Answer from the drawing. Dimensions are ordinates in mm from the lowest x, y and z of the part. A direction names the side the tool comes from. Coordinates: 2 decimals unless noted, no trailing zeros. Loops run counter-clockwise (first coordinate to the right, second up) from the corner with the lowest first, then second, coordinate; pieces in that order, holes last. Notation, with made-up numbers: M 32,44 L 66,44 A16 cw 66,48 Z; hole C 3.25,23.25 d11. An arc over 180 degrees is marked long. Put each result on its own line as item: value.
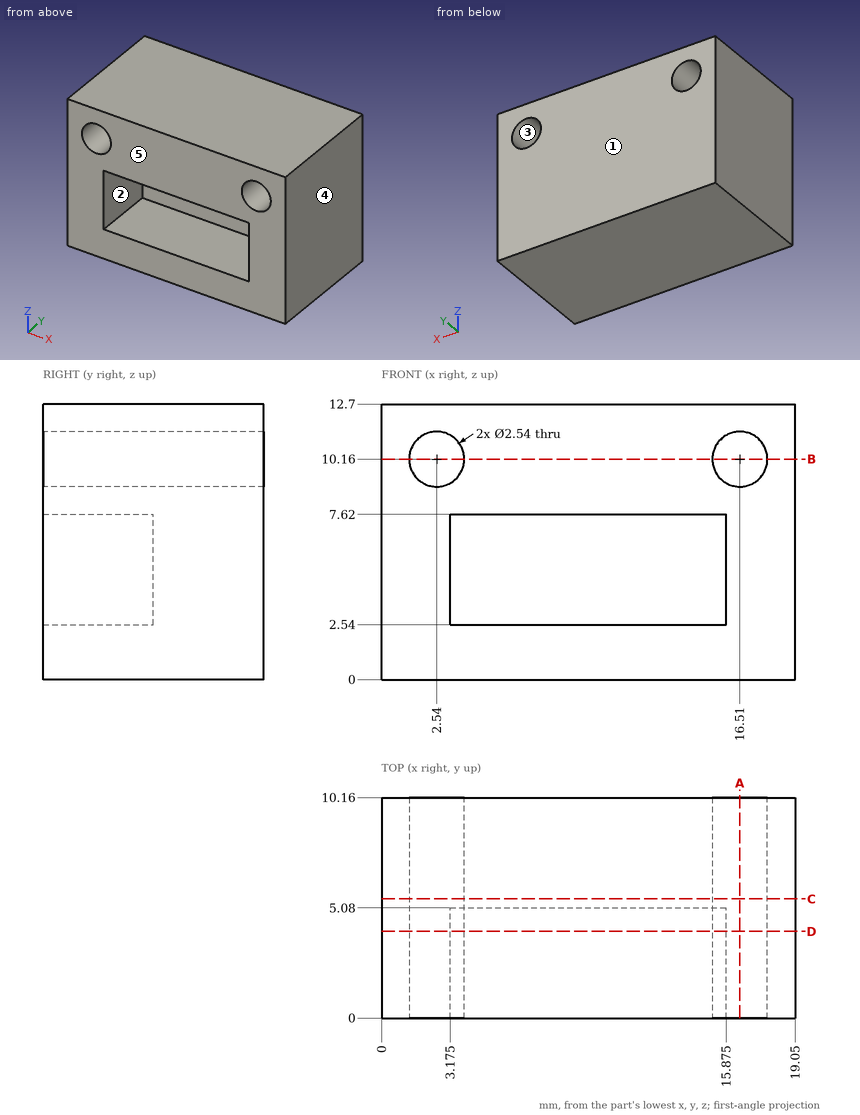
1) Which of the six approach directions +Z, -Z, +X, -X, +Y, -Y give full straight-line access (tool end or side, diameter ignored) to the marked faces 1 and 2?
Answer list:
face 1: +Z, -Z, +X, -X, +Y
face 2: -Y
2) Given pin 1 Ø1.5 at (x, z) = (9, 6) entering from -Y, flat-ended and moving along its own axis, determine where the tip first touches the part or whether it passes through.
Answer list:
pin 1: stops at y = 5.08
3) Find section B-B, the plane z = 10.16. Write down the section's boundary in (x, y), plus the area to 3 significant figures.
Answer list:
outline: M 0,0 L 1.27,0 L 1.27,10.16 L 0,10.16 Z; M 3.81,0 L 15.24,0 L 15.24,10.16 L 3.81,10.16 Z; M 17.78,0 L 19.05,0 L 19.05,10.16 L 17.78,10.16 Z
area: 142 mm^2
4) Find section A-A, the plane x = 16.51. Write down the section's boundary in (y, z), plus the area to 3 significant figures.
Answer list:
outline: M 0,0 L 10.16,0 L 10.16,8.89 L 0,8.89 Z; M 0,11.43 L 10.16,11.43 L 10.16,12.7 L 0,12.7 Z
area: 103 mm^2
5) Determine the mould class of the marked faces 3, 4 and 5 for opening direction X: released by +X, released by -X, zero draft, split by the parting line, or undercut.
Answer list:
face 3: undercut
face 4: released by +X
face 5: zero draft
6) Find section D-D, the plane y = 4. Write down the section's boundary in (x, z) (3 decimals), plus the area to 3 significant figures.
Answer list:
outline: M 0,0 L 19.05,0 L 19.05,12.7 L 0,12.7 Z; hole C 2.54,10.16 d2.54; hole M 3.175,2.54 L 15.875,2.54 L 15.875,7.62 L 3.175,7.62 Z; hole C 16.51,10.16 d2.54
area: 167 mm^2
7) Find section C-C, the plane y = 5.5. Write down the section's boundary in (x, z), plus the area to 3 significant figures.
Answer list:
outline: M 0,0 L 19.05,0 L 19.05,12.7 L 0,12.7 Z; hole C 2.54,10.16 d2.54; hole C 16.51,10.16 d2.54
area: 232 mm^2
8) Straight lines are drawn through the part: line 1 (Z direction, x = 2.54, y = 8); line 2 (Z direction, x = 4, y = 3.25); line 3 (X direction, y = 4.5, z = 9.5). For each, find the intervals that lie inside material, in ascending order. Write a range as [from, to].
Answer list:
line 1: z = [0, 8.89], [11.43, 12.7]
line 2: z = [0, 2.54], [7.62, 12.7]
line 3: x = [0, 1.45], [3.63, 15.42], [17.6, 19.05]
